Job drawing, mm, ordinate dimensions from the low corner. One solid piece. A direction names the side the tool comes from. Round coordinates to 2 decimals unless told otherwise and drop trailing zeros. Order: outer loops, then holes, each group sorted by start corner. A loop starts at its lowest first (then second) coordinate and runs counter-clockwise, first axis right, second up. Notation, with made-up numbers: (41.5, 32.5) -> (80.5, 32.5) arc R27 ccw to (80.5, 52.5) -> close; hole circle Ø2 at (-18.75, 85.25). An arc over 180 degrees is marked (long way). Return JSON: item names as keys, results as strings. Group by question number.
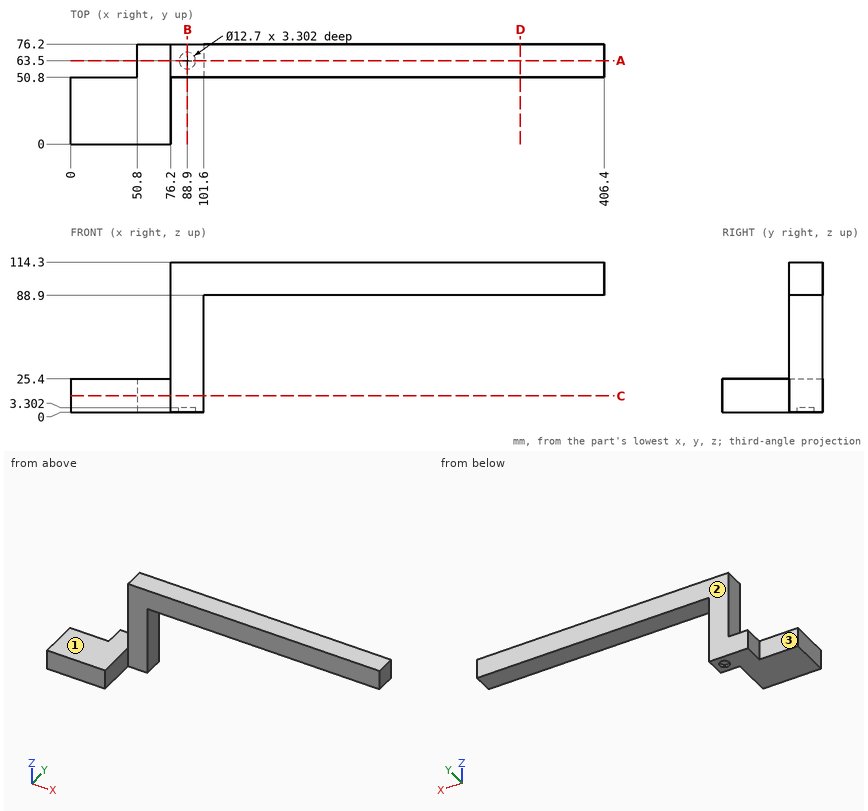
(1) Probe L1, parallel to Y at x = 88.9, z = 1.75; L2, parallel to X at y = 63, z = 1; L3, parallel to Y at x = 101, z = 50. List the from-to ranges inside material, lowest first. Write a range as [from, to].
(2) Saw through at B-B, the plane x = 88.9. List the corners of the cut face in (y, z), and give its area (3 significant figures).
(3) Pin check, flat tips, straight feed: P1, Ø6.5, axis at x = 87, y = 64.5, coming from the -Z side; P2, Ø7.5, axis at y = 65.5, z = 52.5, coming from the -X side; P3, Ø6, axis at y = 45, z = 88.5, coming from the +X side; P4, Ø12.5, axis at x = 21.5, z = 15.5, coming from the +Y side. Stop position of each tip, or through.
(4) Saw through at A-A, the plane y = 63.5. List the corners of the cut face in (x, z).
(5) Saw through at C-C, the plane z = 12.5. List the corners of the cut face in (x, y), and give its area (3 significant figures).
(6) Saw through at D-D, the plane x = 342.5. List the corners of the cut face in (y, z), and give its area (3 significant figures).
(7) Tool access for the marked faces 1, 2 and 3: list every direction of +Z, -Z, +X, -X, +Y, -Y with a clear straight run to the whole face (end or side of a thin tool).
Results are:
{
 "1": {"L1": "y = [50.8, 57.15], [69.85, 76.2]", "L2": "x = [50.8, 82.57], [95.23, 101.6]", "L3": "y = [50.8, 76.2]"},
 "2": {"outline": "(50.8, 0) -> (57.15, 0) -> (57.15, 3.3) -> (69.85, 3.3) -> (69.85, 0) -> (76.2, 0) -> (76.2, 114.3) -> (50.8, 114.3) -> close", "area": "2,860 mm^2"},
 "3": {"P1": "stops at z = 3.3", "P2": "stops at x = 76.2", "P3": "passes through", "P4": "stops at y = 50.8"},
 "4": {"outline": "(50.8, 0) -> (82.55, 0) -> (82.55, 3.3) -> (95.25, 3.3) -> (95.25, 0) -> (101.6, 0) -> (101.6, 88.9) -> (406.4, 88.9) -> (406.4, 114.3) -> (76.2, 114.3) -> (76.2, 25.4) -> (50.8, 25.4) -> close"},
 "5": {"outline": "(0, 0) -> (76.2, 0) -> (76.2, 50.8) -> (101.6, 50.8) -> (101.6, 76.2) -> (50.8, 76.2) -> (50.8, 50.8) -> (0, 50.8) -> close", "area": "5,160 mm^2"},
 "6": {"outline": "(50.8, 88.9) -> (76.2, 88.9) -> (76.2, 114.3) -> (50.8, 114.3) -> close", "area": "645 mm^2"},
 "7": {"face 1": "+Z, -X, +Y, -Y", "face 2": "+Z, -Z, +X, -X, +Y", "face 3": "+Z, -Z, -X, +Y"}
}
